Part print with two shaded views. Sizes in mm from the minimum x, y, z corner. A direction names the side the tool comes from. Give positions to 0.01 mm unless a question says otherwise; leave off trailing zeros. Loops run counter-clockwise (first coordinate to the right, second up) from the corner with the lowest first, then second, coordinate; pieces in that order, holes last. Notation, with made-up numbers: (-6, 58) -> (50, 58) arc R8 cw to (50, 69) -> close; hole circle Ø1 at (64.5, -11). An arc over 180 degrees is marked (long way). One line per question, with ' | ' between items. Start each with the question number.
(1) Slice it at C-C, the plane z = 4.5. Write the cut outline in (x, y), then the cut area to 3 significant figures.
(2) Flat gauge pins, fed straight in: pin 1 Ø1 at (x, z) = (28.5, 1) entering from +Y; pin 2 Ø2.5 at (x, y) = (47, 21.5) entering from +Z; pin 3 Ø1.6 at (y, z) = (9, 4) entering from +X. Where does each tip first touch, or does it go through?
(3) 3-axis set-ups, long thin cutter, end or side, ignore diameter. For the marked faces 1 and 2: which of +Z, -Z, +X, -X, +Y, -Y reach the whole face in a straight line?
(4) Slice it at A-A, the plane x = 3.5. Write the cut outline in (y, z), then the cut area to 3 significant figures.
(5) Slice it at B-B, the plane y = 30. Write the cut outline in (x, z).
(6) Drill centre lines: L1, parallel to X at y = 11.5, z = 1.8; L2, parallel to Y at x = 40, z = 1.85; L3, parallel to X at y = 21, z = 3.95. Where is each one in solid material? Low to high. Write a range as from..to.
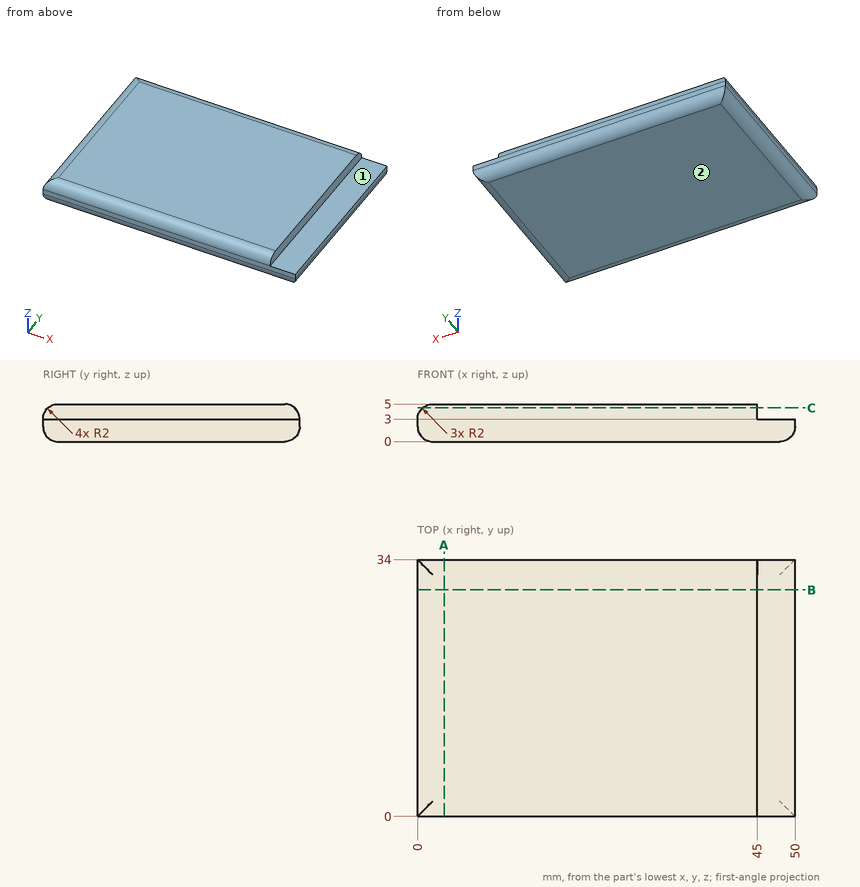
Final values:
1) outline: (0.68, 0.68) -> (45, 0.68) -> (45, 33.32) -> (0.68, 33.32) -> close | area: 1,450 mm2
2) pin 1: y = 33.94 | pin 2: z = 3 | pin 3: x = 45
3) face 1: +Z, +X, +Y, -Y | face 2: -Z, +X, -X, +Y, -Y
4) outline: (0, 2) arc R2 ccw to (2, 0) -> (32, 0) arc R2 ccw to (34, 2) -> (34, 3) arc R2 ccw to (32, 5) -> (2, 5) arc R2 ccw to (0, 3) -> close | area: 167 mm2
5) outline: (0, 2) arc R2 ccw to (2, 0) -> (48, 0) arc R2 ccw to (50, 2) -> (50, 3) -> (45, 3) -> (45, 5) -> (2, 5) arc R2 ccw to (0, 3) -> close
6) L1: 0.01..49.99 | L2: 0.01..33.99 | L3: 0.24..45
